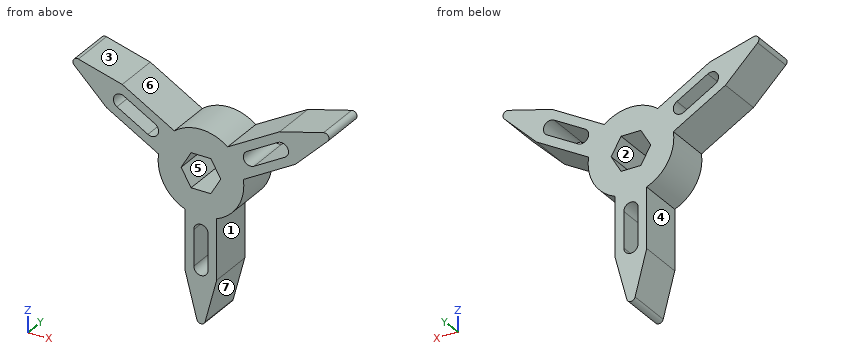
```python
from build123d import *

# Parameters (mm, degrees)
SKETCH1_R           = 30
BOSS_EXTRUDE1_DEPTH = 32


with BuildPart() as part:
    # Sketch1 → Boss-Extrude1 (new body)
    # profile 1 of 4: a face of its own
    with BuildSketch(Plane(origin=(0, 0, 0), x_dir=(1, 0, 0), z_dir=(0, 1, 0))):
        with BuildLine():
            Line((11, 27.910571474), (11, 70))
            Line((11, 70), (2.901151097, 100.763755402))
            ThreePointArc((2.901151097, 100.763755402), (0, 103), (-2.901151097, 100.763755402))
            Line((-2.901151097, 100.763755402), (-11, 70))
            Line((-11, 70), (-11, 27.910571474))
            ThreePointArc((-11, 27.910571474), (0, 30), (11, 27.910571474))
        make_face()
        with BuildLine():
            ThreePointArc((5, 40), (0, 35), (-5, 40))
            Line((-5, 40), (-5, 65))
            ThreePointArc((-5, 65), (0, 70), (5, 65))
            Line((5, 65), (5, 40))
        make_face(mode=Mode.SUBTRACT)
    # profile 2 of 4: a face of its own
    with BuildSketch(Plane(origin=(0, 0, 0), x_dir=(1, 0, 0), z_dir=(0, 1, 0))):
        Circle(SKETCH1_R)
        Polygon((6.92820323, -12), (13.856406461, 0), (6.92820323, 12), (-6.92820323, 12), (-13.856406461, 0), (-6.92820323, -12), align=None, mode=Mode.SUBTRACT)
    # profile 3 of 4: a face of its own
    with BuildSketch(Plane(origin=(0, 0, 0), x_dir=(1, 0, 0), z_dir=(0, 1, 0))):
        with BuildLine():
            Line((66.121778265, -25.473720558), (29.671263931, -4.429006295))
            ThreePointArc((29.671263931, -4.429006295), (25.980762114, -15), (18.671263931, -23.481565179))
            Line((18.671263931, -23.481565179), (55.121778265, -44.526279442))
            Line((55.121778265, -44.526279442), (85.813396411, -52.894348251))
            ThreePointArc((85.813396411, -52.894348251), (89.20061659, -51.5), (88.714547507, -47.869407151))
            Line((88.714547507, -47.869407151), (66.121778265, -25.473720558))
        make_face()
        with BuildLine():
            ThreePointArc((32.141016151, -24.330127019), (30.310889132, -17.5), (37.141016151, -15.669872981))
            Line((37.141016151, -15.669872981), (58.791651246, -28.169872981))
            ThreePointArc((58.791651246, -28.169872981), (60.621778265, -35), (53.791651246, -36.830127019))
            Line((53.791651246, -36.830127019), (32.141016151, -24.330127019))
        make_face(mode=Mode.SUBTRACT)
    # profile 4 of 4: a face of its own
    with BuildSketch(Plane(origin=(0, 0, 0), x_dir=(1, 0, 0), z_dir=(0, 1, 0))):
        with BuildLine():
            ThreePointArc((-18.671263931, -23.481565179), (-25.980762114, -15), (-29.671263931, -4.429006295))
            Line((-29.671263931, -4.429006295), (-66.121778265, -25.473720558))
            Line((-66.121778265, -25.473720558), (-88.714547507, -47.869407151))
            ThreePointArc((-88.714547507, -47.869407151), (-89.20061659, -51.5), (-85.813396411, -52.894348251))
            Line((-85.813396411, -52.894348251), (-55.121778265, -44.526279442))
            Line((-55.121778265, -44.526279442), (-18.671263931, -23.481565179))
        make_face()
        with BuildLine():
            ThreePointArc((-37.141016151, -15.669872981), (-30.310889132, -17.5), (-32.141016151, -24.330127019))
            Line((-32.141016151, -24.330127019), (-53.791651246, -36.830127019))
            ThreePointArc((-53.791651246, -36.830127019), (-60.621778265, -35), (-58.791651246, -28.169872981))
            Line((-58.791651246, -28.169872981), (-37.141016151, -15.669872981))
        make_face(mode=Mode.SUBTRACT)
    extrude(amount=BOSS_EXTRUDE1_DEPTH)


solid = part.part
```
Geometry check sheet. Reference: the model listing, model coordinates, mm. Face numbers are marked on the shaded views. A direction names the side the tool comes from. Give positions to 0.01 mm unless a question says otherwise; leave off trailing zeros. Loops run counter-clockwise (first coordinate to the right, second up) from the corner with the lowest first, then second, coordinate; pieces in that order, holes last. Notation, with made-up numbers: M 19.25,35.25 L 72.25,35.25 A19 ccw 72.25,50.25 Z; hole C 60.25,37.25 d8. An arc over 180 degrees is marked long. Write item = value, one per line. Start each with the question number.
1. Section check C-C, the plane z = 32.5. Enter the section's corners in (x, y), plus the area to 3 significant figures.
2. Draft check along Z on the marked faces 1, 2 and 3. Enter one of: +Z half, -Z half, draft (parallel to the pull), parting line (faces both ways), or undercut.
3. Section check B-B, the plane x = -41. Enter the section's corners in (y, z), plus the area to 3 significant figures.
4. Tool access check on the marked faces 4, 5, 6 and 7. Record the directions out of +Z, -Z, +X, -X, +Y, -Y that give a thin tool (end or side, any length) a straight path to the whole face; none if there is none.
5. Section check D-D, the plane y = 21.5. Give the number of separate pieces and of enclosed holes in the cut face, plus the area to 3 significant figures.
6. Section check A-A, the plane z = -46. Enter the section's corners in (x, y), plus the area to 3 significant figures.
7. Go/stop test with flat-tipped pins: P1, Ø12.5, axis at y = 19, z = -53.5, coming from the +X side; P2, Ø5, axis at x = -4.5, z = -9, coming from the -Y side; P3, Ø1, axis at y = 16.5, z = -45, coming from the -X side; P4, Ø1.5, axis at x = -55, y = 8.5, coming from the +Z side. Record where each tip stops, or that it passes through.
8. Thickness scan on probe 1 along X at (y, z) = (21, 34.5); probe 2 along X at (y, z) = (13, 33); probe 3 along X at (y, z) = (9, -55). Record the ranges inside material, lowest first.
Values follow:
q1.outline = M -73.21,0 L -61.29,0 L -61.29,32 L -73.21,32 Z; M -46.29,0 L -34.29,0 L -34.29,32 L -46.29,32 Z; M 34.29,0 L 46.29,0 L 46.29,32 L 34.29,32 Z; M 61.29,0 L 73.21,0 L 73.21,32 L 61.29,32 Z
q1.area = 1,530 mm^2
q2.face_1 = draft
q2.face_2 = undercut
q2.face_3 = +Z half
q3.outline = M 0,10.97 L 32,10.97 L 32,17.9 L 0,17.9 Z; M 0,29.44 L 32,29.44 L 32,36.37 L 0,36.37 Z
q3.area = 443 mm^2
q4.face_4 = -Z, -X, +Y, -Y
q4.face_5 = +Y, -Y
q4.face_6 = +Z, +Y, -Y
q4.face_7 = -Z, +X, +Y, -Y
q5.separate_pieces = 1
q5.enclosed_holes = 4
q5.area = 5,340 mm^2
q6.outline = M -11,0 L -5,0 L -5,32 L -11,32 Z; M 5,0 L 11,0 L 11,32 L 5,32 Z
q6.area = 384 mm^2
q7.P1 = 11
q7.P2 = through
q7.P3 = -11
q7.P4 = 44.7
q8.probe_1 = -75.23 to -60.87, -49.76 to -37.76, 37.76 to 49.76, 60.87 to 75.23
q8.probe_2 = -73.71 to -61.27, -47.16 to -35.16, 35.16 to 47.16, 61.27 to 73.71
q8.probe_3 = -11 to -5, 5 to 11
